```python
from build123d import *

# Parameters (mm, degrees)
SKETCH_1_R          = 1.25
EXTRUDE_1_DEPTH     = 12
SKETCH_2_R          = 2.34
EXTRUDE_2_DEPTH     = 2.5
CUT_EXTRUDE_1_DEPTH = 1.1
FILLET_1_R          = 0.2


with BuildPart() as part:
    # 草图1 → 凸台-拉伸1 (new body)
    with BuildSketch(Plane(origin=(0, 0, 0), x_dir=(1, 0, 0), z_dir=(0, 1, 0))):
        Circle(SKETCH_1_R)
    extrude(amount=-EXTRUDE_1_DEPTH)

    # 草图2 → 凸台-拉伸2 (add)
    with BuildSketch(Plane(origin=(0, 0, 0), x_dir=(1, 0, 0), z_dir=(0, 1, 0))):
        Circle(SKETCH_2_R)
    extrude(amount=EXTRUDE_2_DEPTH)

    # 草图3 → 切除-拉伸1 (cut)
    with BuildSketch(Plane(origin=(0, 2.5, 0), x_dir=(1, 0, 0), z_dir=(0, 1, 0))):
        Polygon((1.154700538, 0), (0.577350269, 1), (-0.577350269, 1), (-1.154700538, 0), (-0.577350269, -1), (0.577350269, -1), align=None)
    extrude(amount=-CUT_EXTRUDE_1_DEPTH, mode=Mode.SUBTRACT)

    # 圆角1
    fillet_1_edges = [part.edges().sort_by_distance(p)[0] for p in [
        (0.866025404, 1.4, 0.5),
        (1.154700538, 1.95, 0),
        (0, 1.4, 1),
        (0.577350269, 1.95, 1),
        (-0.866025404, 1.4, 0.5),
        (-0.577350269, 1.95, 1),
        (-0.866025404, 1.4, -0.5),
        (-1.154700538, 1.95, 0),
        (0, 1.4, -1),
        (-0.577350269, 1.95, -1),
        (0.866025404, 1.4, -0.5),
        (0.577350269, 1.95, -1),
        (0.866025404, 2.5, 0.5),
        (0.866025404, 2.5, -0.5),
        (0, 2.5, -1),
        (-0.866025404, 2.5, -0.5),
        (-0.866025404, 2.5, 0.5),
        (0, 2.5, 1),
        (-1.25, -12, 0),
        (-2.34, 0, 0),
        (-2.34, 2.5, 0),
    ]]
    fillet(fillet_1_edges, radius=FILLET_1_R)


solid = part.part
```
CAD build for the part. Positions are in the model's coordinates, mm. A direction names the side the tool comes from. Coordinates: 2 decimals unless noted, no trailing zeros. Write each loop counter-clockwise with the first axis right and the second up, starting at its lowest first coordinate (ties: lowest second). Pieces come first, ordered by that corner, then holes. Notation, with made-up numbers: (-33, 38.25) -> (-17, 38.25) arc R22 ccw to (-17, 77.25) -> close; hole circle Ø1 at (57.5, -2.75). An arc over 180 degrees is marked (long way). Use CSV: the item, a comma, the result in double quotes. Start each with the question number.
Item 1: Tool access for faces 4 (the flat face through (0, -12, 0)), 5 (the cylindrical face through (-0.27, -5.82, 1.22)): list every direction of +Z, -Z, +X, -X, +Y, -Y with a clear straight run to the whole face (end or side of a thin tool).
Item 2: Drop flat-ended pins along their axis: P1, Ø1.5, axis at x = -0.5, y = -7, coming from the +Z side; P2, Ø1.3, axis at x = 0, z = 0, coming from the +Y side; P3, Ø1.5, axis at x = -1.5, y = -9, coming from the -Z side. Give the stop position or say it passes through.
Item 3: Two-plate mould, pull along Z, no slides. Class faces 1 (the flat face through (0, 1.4, 0)), 2 (the cylindrical face through (-1.86, 1.24, 1.42)), 3 (the flat face through (1, 0, 1)): +Z half, -Z half, draft (parallel to the pull), parting line (faces both ways), or undercut.
Item 4: Wall check: probe 1 along Y at (x, z) = (0.5, 0.35); probe 2 along X at (y, z) = (-9, -0.05); probe 3 along X at (y, z) = (-4.25, -0.95). Give the ranges that are in metal, low to high.
Item 5: Band-saw the part on B-B, the plane y = -0.75. Write the cut outline in (x, z).
Item 6: Band-saw the part on A-A, the plane x = 0. Write the cut outline in (y, z).
Response values:
1,face 4,"+Z, -Z, +X, -X, -Y"
1,face 5,"-Y"
2,P1,"stops at z = 1.25"
2,P2,"stops at y = 1.4"
2,P3,"stops at z = -1"
3,face 1,"undercut"
3,face 2,"parting line"
3,face 3,"draft"
4,probe 1,"y = -12 to 1.4"
4,probe 2,"x = -1.25 to 1.25"
4,probe 3,"x = -0.81 to 0.81"
5,outline,"circle Ø2.5 at (0, 0)"
6,outline,"(-12, -1.05) arc R0.2 ccw to (-11.8, -1.25) -> (0, -1.25) -> (0, -2.14) arc R0.2 ccw to (0.2, -2.34) -> (2.3, -2.34) arc R0.2 ccw to (2.5, -2.14) -> (2.5, -1.2) arc R0.2 ccw to (2.3, -1) -> (1.6, -1) arc R0.2 cw to (1.4, -0.8) -> (1.4, 0.8) arc R0.2 cw to (1.6, 1) -> (2.3, 1) arc R0.2 ccw to (2.5, 1.2) -> (2.5, 2.14) arc R0.2 ccw to (2.3, 2.34) -> (0.2, 2.34) arc R0.2 ccw to (0, 2.14) -> (0, 1.25) -> (-11.8, 1.25) arc R0.2 ccw to (-12, 1.05) -> close"
